from build123d import *

# Parameters (mm, degrees)
SKETCH_1_W      = 45.450980392
SKETCH_1_H      = 61
SKETCH_1_R      = 1.5
EXTRUDE_1_DEPTH = 1.6
FILLET_1_R      = 5


with BuildPart() as part:
    # 草图1 → 凸台-拉伸1 (new body)
    with BuildSketch(Plane.XY):
        Rectangle(SKETCH_1_W, SKETCH_1_H)
        with Locations((19, -25.5)):
            Circle(SKETCH_1_R, mode=Mode.SUBTRACT)
        with Locations((-19, -25.5)):
            Circle(SKETCH_1_R, mode=Mode.SUBTRACT)
        with Locations((-19, 25.5)):
            Circle(SKETCH_1_R, mode=Mode.SUBTRACT)
        with Locations((19, 25.5)):
            Circle(SKETCH_1_R, mode=Mode.SUBTRACT)
        with Locations((-8.227241336, -4.75)):
            Circle(SKETCH_1_R, mode=Mode.SUBTRACT)
        with Locations((8.227241336, -4.75)):
            Circle(SKETCH_1_R, mode=Mode.SUBTRACT)
        with Locations((0, 9.5)):
            Circle(SKETCH_1_R, mode=Mode.SUBTRACT)
    extrude(amount=EXTRUDE_1_DEPTH)

    # 圆角1
    fillet_1_edges = [part.edges().sort_by_distance(p)[0] for p in [
        (22.725490196, -30.5, 0.8),
        (-22.725490196, -30.5, 0.8),
        (-22.725490196, 30.5, 0.8),
        (22.725490196, 30.5, 0.8),
    ]]
    fillet(fillet_1_edges, radius=FILLET_1_R)


solid = part.part
Source: CAD feature listing. Evaluate the final solid. Frame: model axes, mm. Coordinates: 2 decimals unless noted, no trailing zeros. Order: outer loops, then holes, each group sorted by start corner. A loop starts at its lowest first (then second) coordinate and runs counter-clockwise, first axis right, second up. Notation, with made-up numbers: M -26,89.5 L 2,89.5 A23 cw 2,98.5 Z; hole C -22,35 d11. An arc over 180 degrees is marked long. Write each question's results on one line, items separated by ' | '. Start each with the question number.
1. Draft query along Y for faces 1 (the face through (-22.725, 0, 1)), 2 (the face through (-20.11, -24.49, 0.79)), 3 (the face through (0, 30.5, 1)), 4 (the face through (21.222, -29.074, 0.811)). Return one class per face: +Y half, -Y half, draft (parallel to the pull), parting line (faces both ways), or undercut.
2. Material intervals for L1, parallel to Y at x = 0, z = 0.9; L2, parallel to Y at x = 19.5, z = 1; L3, parallel to Y at x = -20, z = 0.4, sorted ascending.
3. Pin query (flat end, axial travel): pin 1 (1.8 mm diameter, centred on x = -8.23, y = -4.75, fed in from -Z). Return the tip coordinate at first contact, or that it passes through.
4. Section C-C, the plane z = 1.2. Return the cut outline in (x, y), then the cut area to 3 significant figures.
5. Section A-A, the plane y = 9.5. Return the cut outline in (x, z).
6. Section B-B, the plane x = 0. Return the cut outline in (y, z).
7. Section D-D, the plane x = -19. Return the cut outline in (y, z), then the cut area to 3 significant figures.
Solution:
1) face 1: draft | face 2: undercut | face 3: +Y half | face 4: -Y half
2) L1: -30.5 to 8, 11 to 30.5 | L2: -30.17 to -26.91, -24.09 to 24.09, 26.91 to 30.17 | L3: -29.95 to -26.62, -24.38 to 24.38, 26.62 to 29.95
3) pin 1: through
4) outline: M -22.73,-25.5 A5 ccw -17.73,-30.5 L 17.73,-30.5 A5 ccw 22.73,-25.5 L 22.73,25.5 A5 ccw 17.73,30.5 L -17.73,30.5 A5 ccw -22.73,25.5 Z; hole C -19,-25.5 d3; hole C -19,25.5 d3; hole C -8.23,-4.75 d3; hole C 0,9.5 d3; hole C 8.23,-4.75 d3; hole C 19,-25.5 d3; hole C 19,25.5 d3 | area: 2,700 mm²
5) outline: M -22.73,0 L -1.5,0 L -1.5,1.6 L -22.73,1.6 Z; M 1.5,0 L 22.73,0 L 22.73,1.6 L 1.5,1.6 Z
6) outline: M -30.5,0 L 8,0 L 8,1.6 L -30.5,1.6 Z; M 11,0 L 30.5,0 L 30.5,1.6 L 11,1.6 Z
7) outline: M -30.33,0 L -27,0 L -27,1.6 L -30.33,1.6 Z; M -24,0 L 24,0 L 24,1.6 L -24,1.6 Z; M 27,0 L 30.33,0 L 30.33,1.6 L 27,1.6 Z | area: 87.5 mm²
